Geometry: final body of the model. Coordinates: model frame, mm. Face numbers are marked on the shaded views. A direction names the side the tool comes from. Coordinates: 2 decimals unless noted, no trailing zeros. Loops run counter-clockwise (first coordinate to the right, second up) from the corner with the lowest first, then second, coordinate; pieces in that order, holes last. Notation, with made-up numbers: (75, 66.5) - (99, 66.5) arc R8 cw to (99, 71.5) - close; hole circle Ø9 at (49.5, 29.5). An arc over 180 degrees is marked (long way). Answer in a Markdown table with one row per item.
from build123d import *

# Parameters (mm, degrees)
EXTRUDE_1_DEPTH     = 20
SKETCH_2_R          = 2
CUT_EXTRUDE_1_DEPTH = 6
SKETCH_3_R          = 1.95
EXTRUDE_2_DEPTH     = 5


with BuildPart() as part:
    # 草图1 → 凸台-拉伸1 (new body)
    with BuildSketch(Plane(origin=(0, 0, 0), x_dir=(1, 0, 0), z_dir=(0, 1, 0))):
        with BuildLine():
            Line((-15, 0), (15, 0))
            ThreePointArc((15, 0), (0, -15), (-15, 0))
        make_face()
    extrude(amount=EXTRUDE_1_DEPTH)

    # 草图2 → 切除-拉伸1 (cut)
    with BuildSketch(Plane(origin=(0, 20, 0), x_dir=(1, 0, 0), z_dir=(0, 1, 0))):
        with Locations(Location((-5, -5, 0), (0, 0, 270))):
            Circle(SKETCH_2_R)
        with Locations(Location((5, -5, 0), (0, 0, 90))):
            Circle(SKETCH_2_R)
    extrude(amount=-CUT_EXTRUDE_1_DEPTH, mode=Mode.SUBTRACT)

    # 草图3 → 凸台-拉伸2 (add)
    with BuildSketch(Plane.XZ):
        with Locations(Location((5, 5, 0), (0, 0, 90))):
            Circle(SKETCH_3_R)
        with Locations(Location((-5, 5, 0), (0, 0, 90))):
            Circle(SKETCH_3_R)
    extrude(amount=EXTRUDE_2_DEPTH)


solid = part.part
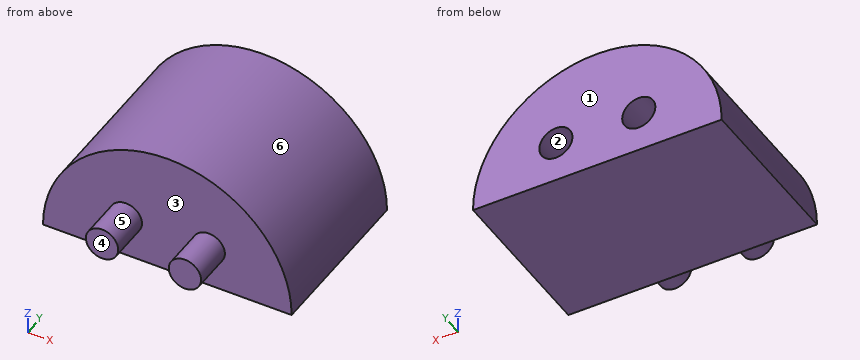
(1) Cut plane C-C on z = 9. Output: boundary loops of the cut face in (x, y).
Verdict:
| item | result |
|---|---|
| outline | (-12, 0) - (12, 0) - (12, 20) - (-12, 20) - close |
(2) Access query for the marked faces 1, 2 and 3. Directions: +Z, -Z, +X, -X, +Y, -Y. A direction counts if a zero-diameter tool reaches every point of the face in a straight line with its end or side. Return the directions, or none.
Verdict:
| item | result |
|---|---|
| face 1 | +Z, -Z, +X, -X, +Y |
| face 2 | +Y |
| face 3 | -Y |
(3) Cut plane D-D on y = 5.75. Output: boundary loops of the cut face in (x, z).
Verdict:
| item | result |
|---|---|
| outline | (-15, 0) - (15, 0) arc R15 ccw to start |
(4) Ray query, probe 1 along X at (y, z) = (17.2, 5); probe 2 along Y at (x, z) = (6.5, 4.5); probe 3 along Z at (x, y) = (5, 17.05). Return the intervals inside material, ascending.
Verdict:
| item | result |
|---|---|
| probe 1 | x = -14.14 to -7, -3 to 3, 7 to 14.14 |
| probe 2 | y = -5 to 14 |
| probe 3 | z = 0 to 3, 7 to 14.14 |
(5) First-contact query: pin 1 Ø1.2 at (x, z) = (6, 5.5) entering from +Y; pin 2 Ø1 at (y, z) = (4, 5.5) entering from +X; pin 3 Ø4.5 at (x, z) = (0, 6) entering from -Y; pin 4 Ø2 at (x, z) = (-4.5, 6) entering from +Y. Flat tips, straight axial feed; report the tip coordinate or a pass-through.
Verdict:
| item | result |
|---|---|
| pin 1 | stops at y = 14 |
| pin 2 | stops at x = 14.14 |
| pin 3 | stops at y = 0 |
| pin 4 | stops at y = 20 |
(6) Cut plane B-B on x = 5. Output: boundary loops of the cut face in (y, z), then the cut area to 3 significant figures.
Verdict:
| item | result |
|---|---|
| outline | (-5, 3.05) - (0, 3.05) - (0, 0) - (20, 0) - (20, 3) - (14, 3) - (14, 7) - (20, 7) - (20, 14.14) - (0, 14.14) - (0, 6.95) - (-5, 6.95) - close |
| area | 278 mm² |
(7) Pull-direction query (X, two-part tool) for the marked faces 4, 5 and 6; classes: pulls with the +X half, pulls with the -X half, needs draft (parallel to the pull), parting line crosses it, or undercut.
Verdict:
| item | result |
|---|---|
| face 4 | needs draft |
| face 5 | undercut |
| face 6 | parting line crosses it |
(8) Cut plane A-A on y = 17.25. Output: boundary loops of the cut face in (x, z), then the cut area to 3 significant figures.
Verdict:
| item | result |
|---|---|
| outline | (-15, 0) - (15, 0) arc R15 ccw to start; hole circle Ø4 at (-5, 5); hole circle Ø4 at (5, 5) |
| area | 328 mm² |
